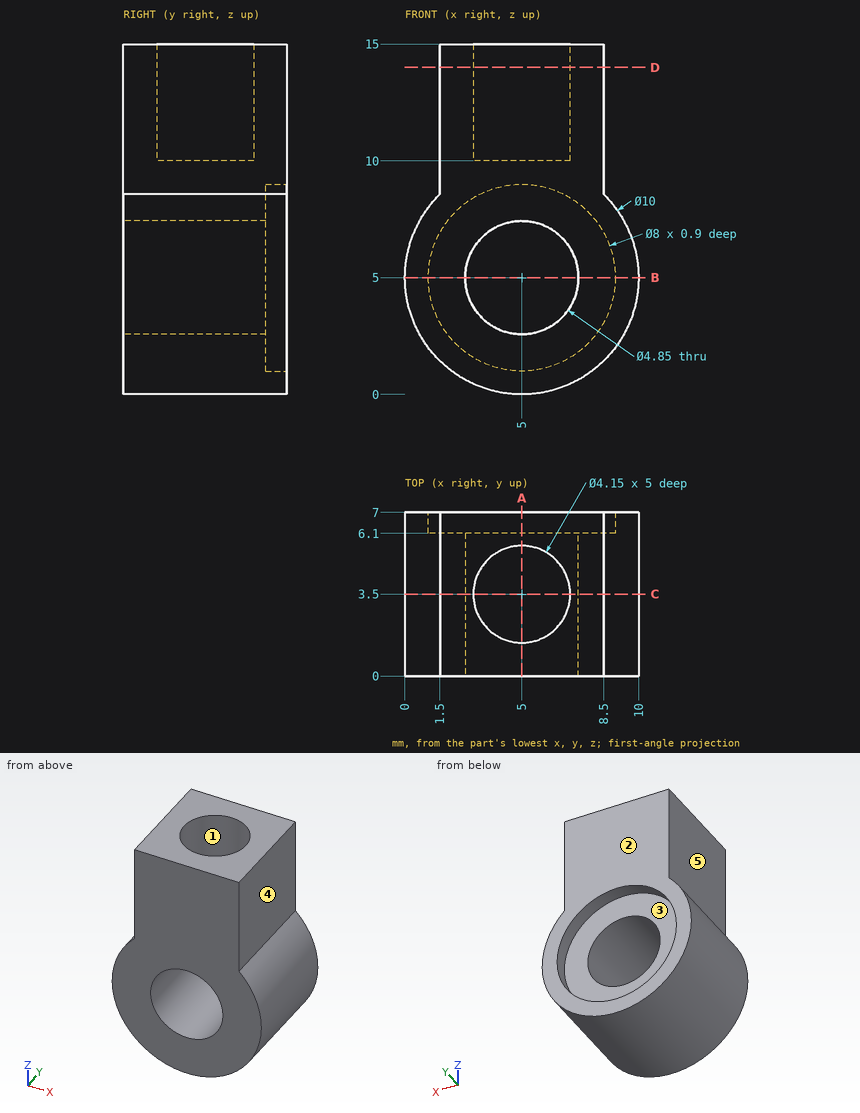
Answer from the drawing. Dimensions are ordinates in mm from the lowest x, y and z of the part. A direction names the side the tool comes from. Give positions to 0.01 mm unless a question says otherwise; leave off trailing zeros. Loops run counter-clockwise (first coordinate to the right, second up) from the corner with the lowest first, then second, coordinate; pieces in that order, holes last.
Item 1: Each of these flat-tipped pins is pushed along its axis until it touches: pin 1 Ø4.5 at (x, z) = (5, 5) entering from -Y; pin 2 Ø1.9 at (y, z) = (5, 12.5) entering from +X; pin 3 Ø2 at (y, z) = (2.5, 2.5) entering from +X; pin 4 Ø1 at (y, z) = (6, 10) entering from -X. Where does it stop, or does it pass through?
Item 2: The part is cut by section D-D (z = 14). Write down the section's boundary in (x, y) (3 decimals).
Item 3: Find the intervals of material crossed by line 1 along X through (y, z) = (6.5, 5); line 2 along X through (y, z) = (4.75, 5) (3 decimals); line 3 along Y through (x, z) = (3, 1.75), in increasing order.
Item 4: The mould has two halves that part along X. Classify the marked faces 3, 4 and 5: released by +X, released by -X, zero draft, split by the parting line, or undercut.
Item 5: For the marked faces 1 and 2, determine the directions among +Z, -Z, +X, -X, +Y, -Y from which every point of the face is accessible in a straight line to the end or side of a thin tool.
Item 6: The part is cut by section B-B (z = 5). Write down the section's boundary in (x, y) (3 decimals), and give its area (3 significant figures).
Item 7: The part is cut by section A-A (x = 5). Write down the section's boundary in (y, z) (3 decimals), and give its area (3 significant figures).
Item 8: The part is cut by section C-C (y = 3.5). Write down the section's boundary in (x, z) (3 decimals), and give its area (3 significant figures).
Taken from the geometry:
1. pin 1: passes through
1. pin 2: stops at x = 8.5
1. pin 3: stops at x = 9.77
1. pin 4: stops at x = 1.5
2. outline: (1.5, 0) - (8.5, 0) - (8.5, 7) - (1.5, 7) - close; hole circle Ø4.15 at (5, 3.5)
3. line 1: x = 0 to 1, 9 to 10
3. line 2: x = 0 to 2.575, 7.425 to 10
3. line 3: y = 0 to 6.1
4. face 3: undercut
4. face 4: released by +X
4. face 5: released by -X
5. face 1: +Z
5. face 2: +Z, -Z, +X, -X, +Y
6. outline: (0, 0) - (2.575, 0) - (2.575, 6.1) - (1, 6.1) - (1, 7) - (0, 7) - close; (7.425, 0) - (10, 0) - (10, 7) - (9, 7) - (9, 6.1) - (7.425, 6.1) - close
6. area: 33.2 mm2
7. outline: (0, 0) - (7, 0) - (7, 1) - (6.1, 1) - (6.1, 2.575) - (0, 2.575) - close; (0, 7.425) - (6.1, 7.425) - (6.1, 9) - (7, 9) - (7, 15) - (5.575, 15) - (5.575, 10) - (1.425, 10) - (1.425, 15) - (0, 15) - close
7. area: 47.5 mm2
8. outline: (1.5, 8.571) arc R5 ccw (long way) to (8.5, 8.571) - (8.5, 15) - (7.075, 15) - (7.075, 10) - (2.925, 10) - (2.925, 15) - (1.5, 15) - close; hole circle Ø4.85 at (5, 5)
8. area: 77.4 mm2
